Verification items for the finished model (mm, model axes). A direction names the side the tool comes from. Round coordinates to 2 decimals unless told otherwise and drop trailing zeros. Write each loop counter-clockwise with the first axis right and the second up, starting at its lowest first coordinate (ties: lowest second). Pieces come first, ordered by that corner, then holes. Notation, with made-up numbers: M 53,27.5 L 84,27.5 A21 ccw 84,53.5 Z; hole C 83,14 d5. An arc over 180 degrees is marked long. One line per item, written item: value. Start each with the question number.
Item 1: Tool access check on faces 5 (the face through (5, -25.4, 13)), 6 (the face through (12.177, -12.522, 22.937)). Record the directions out of +Z, -Z, +X, -X, +Y, -Y that give a thin tool (end or side, any length) a straight path to the whole face; none if there is none.
Item 2: Draft check along Z on faces 1 (the face through (-20.95, -38, 13)), 2 (the face through (-9, -25, -18.914)), 3 (the face through (18, -38, -6.214)), 4 (the face through (-55.71, -25.044, 40.466)). Enter one of: +Z half, -Z half, draft (parallel to the pull), parting line (faces both ways), or undercut.
Item 3: Gauge pin test, flat ends, axial feed: pin 1 (8 mm diameter, centred on y = -15.5, z = 37.5, fed in from -X); pin 2 (7.5 mm diameter, centred on y = -41, z = 12, fed in from +X); pin 3 (20.5 mm diameter, centred on x = 13, y = -37, fed in from +Z). Record the tip position at first contact, or that the pin passes through.
Item 4: Thickness scan on probe 1 along X at (y, z) = (-10.5, -11); probe 2 along Z at (x, y) = (10, -43); probe 3 along X at (y, z) = (-27, 5). Record the ranges inside material, lowest first. Write a range as from..to.
Item 5: Section check B-B, the plane y = -3. Record the cut outline in (x, z), then the cut area to 3 significant figures.
Item 6: Section check D-D, the plane x = -5. Record the cut outline in (y, z), then the cut area to 3 significant figures.
Item 7: Section check C-C, the plane x = -39.5. Record the cut outline in (y, z).
Item 8: Section check A-A, the plane z = 33.5. Record the cut outline in (x, y), then the cut area to 3 significant figures.
from build123d import *

# Parameters (mm, degrees)
F0_R     = 12.7
F1_DEPTH = 25.4
F2_R     = 12.7
F3_DEPTH = 25.4
F4_R     = 12.7


with BuildPart() as f1:
    # F0 (on Front) → F1 (new body)
    with BuildSketch(Plane.XZ):
        with BuildLine():
            Line((55.243076, -6.21413), (-32.111921, 52.916597))
            ThreePointArc((-32.111921, 52.916597), (-58.254618, 54.319874), (-71.749997, 31.88587))
            Line((-71.749997, 31.88587), (-71.756924, -18.91413))
            Line((-71.756924, -18.91413), (55.243076, -18.91413))
            Line((55.243076, -18.91413), (55.243076, -6.21413))
        make_face()
        with Locations((-46.349997, 31.882406)):
            Circle(F0_R, mode=Mode.SUBTRACT)
    extrude(amount=F1_DEPTH)

    # F2 (on face) → F3 (join)
    with BuildSketch(Plane.XZ.offset(25.4)):
        with BuildLine():
            Line((-20.949997, -6.21413), (-20.949997, 31.882406))
            ThreePointArc((-20.949997, 31.882406), (-23.91334, 43.788557), (-32.111921, 52.916597))
            ThreePointArc((-32.111921, 52.916597), (-58.254618, 54.319874), (-71.749997, 31.88587))
            Line((-71.749997, 31.88587), (-71.755192, -6.21413))
            Line((-71.755192, -6.21413), (-71.756058, -12.56413))
            Line((-71.756058, -12.56413), (-71.756924, -18.91413))
            Line((-71.756924, -18.91413), (55.243076, -18.91413))
            Line((55.243076, -18.91413), (55.243076, -6.21413))
            Line((55.243076, -6.21413), (-20.949997, -6.21413))
        make_face()
        with Locations((-46.349997, 31.882406)):
            Circle(F2_R, mode=Mode.SUBTRACT)
    extrude(amount=F3_DEPTH)

    # F4
    f4_edges = [f1.edges().sort_by_distance(p)[0] for p in [
        (55.243076, -50.8, -12.56413),
    ]]
    fillet(f4_edges, radius=F4_R)


solid = f1.part
Response values:
1. face 5: +Z, +X, -Y
1. face 6: +Z, +X, +Y, -Y
2. face 1: draft
2. face 2: -Z half
2. face 3: +Z half
2. face 4: undercut
3. pin 1: stops at x = -71.7
3. pin 2: stops at x = -20.95
3. pin 3: stops at z = -6.21
4. probe 1: x = -71.76..55.24
4. probe 2: z = -18.91..-6.21
4. probe 3: x = -71.75..-20.95
5. outline: M -71.76,-18.91 L 55.24,-18.91 L 55.24,-6.21 L -32.11,52.92 A25.4 ccw -71.75,31.89 Z; hole C -46.35,31.88 d25.4
5. area: 6,050 mm2
6. outline: M -50.8,-18.91 L 0,-18.91 L 0,34.56 L -25.4,34.56 L -25.4,-6.21 L -50.8,-6.21 Z
6. area: 1,680 mm2
7. outline: M -50.8,-18.91 L 0,-18.91 L 0,21.19 L -50.8,21.19 Z; M -50.8,42.58 L 0,42.58 L 0,56.34 L -50.8,56.34 Z
8. outline: M -71.7,-50.8 L -58.95,-50.8 L -58.95,0 L -71.7,0 Z; M -33.75,-50.8 L -21,-50.8 L -21,-25.4 L -3.43,-25.4 L -3.43,0 L -33.75,0 Z
8. area: 1,740 mm2
